Model file for the job. Use its own axes, mm. Face numbers are marked on the shaded views. A direction names the side the tool comes from. Coordinates: 2 decimals unless noted, no trailing zeros. Order: outer loops, then holes, each group sorted by start corner. A loop starts at its lowest first (then second) coordinate and runs counter-clockwise, first axis right, second up. Notation, with made-up numbers: (66.5, 66.25) -> (112.5, 66.25) arc R18 ccw to (112.5, 101.25) -> close; hole circle Ø5 at (68, 85.25). An arc over 180 degrees is marked (long way). Return JSON: item names as keys, results as strings. Group by question number.
1) Pull direction Y, two halves, no side cores. Call the marked faces 4, 5 and 6: +Y half, -Y half, draft (parallel to the pull), parting line (faces both ways), or undercut.
2) Which spindle directions (+Z, -Z, +X, -X, +Y, -Y) get a long thin tool onto all of the face, cutting with end or side? Do the marked faces 1, 2 and 3. Say none if no direction does.
3) Flat gauge pins, fed straight in: pin 1 (4 mm diameter, centred on y = 16, z = 26, fed in from -X); pin 2 (6 mm diameter, centred on y = -6, z = 16.5, fed in from -X); pin 3 (12 mm diameter, centred on y = -14, z = 11.5, fed in from +X). Where does each tip first touch, or does it go through?
4) Cut at D-D (z = 15). Write the cut outline in (x, y).
5) Probe line 1 (Y direction, x = 3.5, z = 16.5); line 2 (Y direction, x = 17, z = 32); line 3 (X direction, y = -2, z = 11.5). List the from-to ranges inside material, lowest first.
6) Cut at A-A (y = 0). Write the cut outline in (x, z).
from build123d import *

# Parameters (mm, degrees)
SKETCH_R           = 31
PAD_DEPTH          = 40
SKETCH001_R        = 22.2
POCKET_DEPTH       = 20
SKETCH002_R        = 1.5
PAD001_DEPTH       = 25
POLARPATTERN_COUNT = 16
SKETCH003_W        = 9.8
SKETCH003_H        = 9.8
POCKET001_DEPTH    = 40.001


with BuildPart() as part:
    # Sketch → Pad (new body)
    with BuildSketch(Plane.XY):
        Circle(SKETCH_R)
    extrude(amount=PAD_DEPTH)

    # Sketch001 → Pocket (cut)
    with BuildSketch(Plane.XY.offset(40)):
        Circle(SKETCH001_R)
    extrude(amount=-POCKET_DEPTH, mode=Mode.SUBTRACT)

    # Sketch002 → Pad001 (new body)
    with BuildSketch(Plane.XY.offset(40)):
        with Locations((0, 22.2)):
            Circle(SKETCH002_R)
    pad001 = extrude(amount=-PAD001_DEPTH)

    # PolarPattern: Pad001 ×16 about axis
    polarpattern_axis = Axis((0, 0, 40), (0, 0, 1))
    for i in range(1, POLARPATTERN_COUNT):
        add(pad001.rotate(polarpattern_axis, i * 360 / POLARPATTERN_COUNT))

    # Sketch003 → Pocket001 (cut, through all)
    with BuildSketch(Plane(origin=(0, 0, 0), x_dir=(1, 0, 0), z_dir=(0, 0, -1))):
        Rectangle(SKETCH003_W, SKETCH003_H)
    extrude(amount=-POCKET001_DEPTH, mode=Mode.SUBTRACT)


solid = part.part
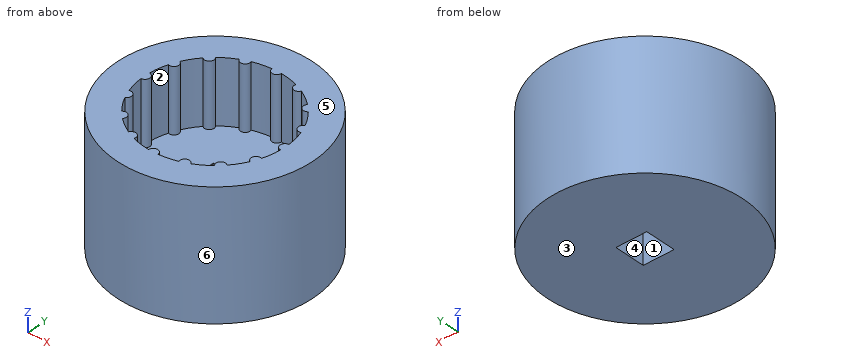
Answers below:
{
 "1": {"face 4": "undercut", "face 5": "draft", "face 6": "parting line"},
 "2": {"face 1": "+Z, -Z", "face 2": "+Z", "face 3": "-Z, +X, -X, +Y, -Y"},
 "3": {"pin 1": "stops at x = -27.66", "pin 2": "stops at x = -30.85", "pin 3": "stops at x = 29.95"},
 "4": {"outline": "circle Ø62 at (0, 0); hole (-4.9, -4.9) -> (4.9, -4.9) -> (4.9, 4.9) -> (-4.9, 4.9) -> close"},
 "5": {"line 1": "y = -30.8 to -4.9, 4.9 to 30.8", "line 2": "y = -25.92 to -14.28, 14.28 to 25.92", "line 3": "x = -30.94 to -4.9, 4.9 to 30.94"},
 "6": {"outline": "(-31, 0) -> (-4.9, 0) -> (-4.9, 20) -> (-20.7, 20) -> (-20.7, 40) -> (-31, 40) -> close; (4.9, 0) -> (31, 0) -> (31, 40) -> (20.7, 40) -> (20.7, 20) -> (4.9, 20) -> close"}
}
